Verification items for this drawing (mm, ordinates from the low corner). A direction names the side the tool comes from. Round coordinates to 2 decimals unless told otherwise and drop trailing zeros. Order: outer loops, then holes, each group sorted by start corner. A loop starts at its lowest first (then second) coordinate and runs counter-clockwise, first axis right, second up. Notation, with made-up numbers: (-29, 37.25) - (-3, 37.25) arc R15 ccw to (-3, 62.25) - close; hole circle Ø3 at (-25, 17.5). An arc over 180 degrees is marked (long way). One line per question, with ' | ' between items. Start each with the question number.
Q1. Material ranges on line 1 along Y through (x, z) = (5.75, 1.1); line 2 along Z through (x, y) = (16, 23.5); line 3 along Y through (x, z) = (14.25, 2.4), recorded low to high.
Q2. Gauge pin test, flat ends, axial feed: P1, Ø4, axis at x = 4.5, y = 18, coming from the +Z side; P2, Ø3, axis at x = 17.5, z = 3, coming from the -Y side; P3, Ø1.2, axis at y = 2.5, z = 1, coming from the +X side. Record the tip position at first contact, or that the pin passes through.
Q3. Mould release check, pull along Y, two halves, no side actions. Record for the marked faces 1, 2, 3 and 4: +Y half, -Y half, draft (parallel to the pull), parting line (faces both ways), or undercut.
Q4. Sectioned sample at C-C, the plane z = 4.2. Enter the section's corners in (x, y).
Q5. Tool access check on the marked faces 5 and 6. Record the directions out of +Z, -Z, +X, -X, +Y, -Y that give a thin tool (end or side, any length) a straight path to the whole face; none if there is none.
Q6. Sectioned sample at A-A, the plane y = 19.25. Enter the section's corners in (x, z).
Q7. Sectioned sample at B-B, the plane x = 5.75. Enter the section's corners in (y, z).
Q8. Sectioned sample at D-D, the plane y = 5.75. Enter the section's corners in (x, z), then the cut area to 4 significant figures.
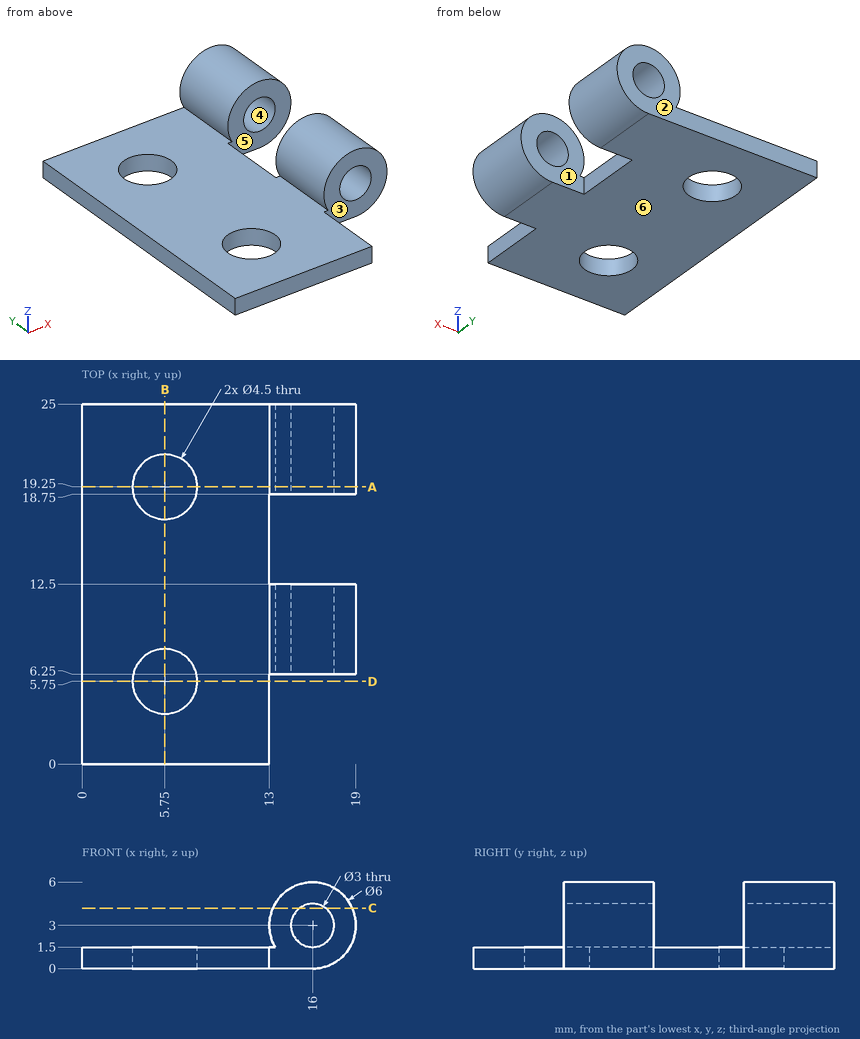
Determined:
1) line 1: y = 0 to 3.5, 8 to 17, 21.5 to 25 | line 2: z = 0 to 1.5, 4.5 to 6 | line 3: y = 6.25 to 12.5, 18.75 to 25
2) P1: stops at z = 1.5 | P2: stops at y = 6.25 | P3: stops at x = 13
3) face 1: undercut | face 2: +Y half | face 3: -Y half | face 4: draft
4) outline: (13.25, 6.25) - (15.1, 6.25) - (15.1, 12.5) - (13.25, 12.5) - close; (13.25, 18.75) - (15.1, 18.75) - (15.1, 25) - (13.25, 25) - close; (16.9, 6.25) - (18.75, 6.25) - (18.75, 12.5) - (16.9, 12.5) - close; (16.9, 18.75) - (18.75, 18.75) - (18.75, 25) - (16.9, 25) - close
5) face 5: +Z, -Z, +X | face 6: -Z, +X, -X, +Y, -Y
6) outline: (0, 0) - (3.5, 0) - (3.5, 1.5) - (0, 1.5) - close; (8, 0) - (16, 0) arc R3 ccw (long way) to (13.4, 1.5) - (8, 1.5) - close; hole circle Ø3 at (16, 3)
7) outline: (0, 0) - (3.5, 0) - (3.5, 1.5) - (0, 1.5) - close; (8, 0) - (17, 0) - (17, 1.5) - (8, 1.5) - close; (21.5, 0) - (25, 0) - (25, 1.5) - (21.5, 1.5) - close
8) outline: (0, 0) - (3.5, 0) - (3.5, 1.5) - (0, 1.5) - close; (8, 0) - (13, 0) - (13, 1.5) - (8, 1.5) - close | area: 12.75 mm2
